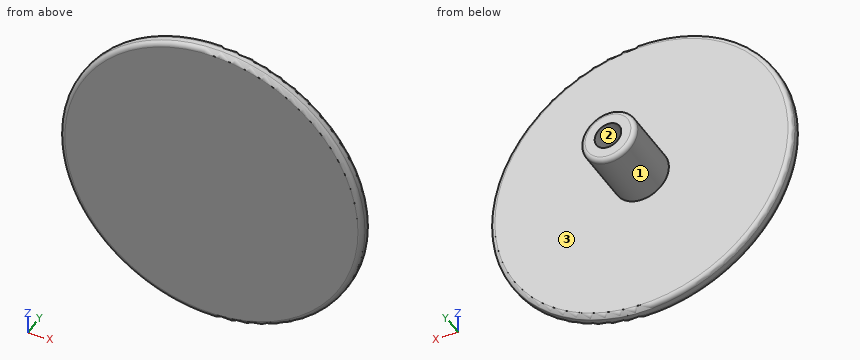
Autodesk Fusion 360 part; units mm, degrees
sketch "Sketch1" plane through (0, 0, 0) normal (0, 1, 0) x (1, 0, 0)
  circle A0 centre (0, 0) radius 16.5
  dimension "d1" = 33
extrude "Extrude1" add sketch "Sketch1" along normal blind 1.5
sketch "Sketch2" plane through (0, 1.5, 0) normal (0, 1, 0) x (-1, 0, 0)
  circle A0 centre (0, 0) radius 16.5
  circle A1 centre (0, 0) radius 3
  circle A2 centre (0, 0) radius 1.45
  dimension "d4" = 6
  dimension "d5" = 2.9
extrude "Extrude2" add sketch "Sketch2" along normal blind 7 contours A1
fillet "Fillet1" radius 0.5 3 edges at (-15.3834, 0, 5.9667) (-15.3834, 1.5, 5.9667) (2.797, 8.5, -1.0848)
The listing builds one solid part. Answer for the finished solid, in the listing's coordinates (mm). Face numbers are marked on the shaded views. Round coordinates to 2 decimals unless told otherwise and drop trailing zeros. Loops run counter-clockwise (first coordinate to the right, second up) from the corner with the lowest first, then second, coordinate; pieces in that order, holes last. Notation, with made-up numbers: (-25.5, 67) - (-20.5, 67) arc R16 ccw to (-20.5, 98) - close; hole circle Ø8 at (61.25, 60). An arc over 180 degrees is marked (long way). Return JSON: item names as keys, results as strings. Group by question number.
1. The part is cut by section B-B on z = 0. Determine the outline of the cut face in (x, y).
2. Each of these flat-tipped pins is pushed along its axis until it touches: P1, Ø5, axis at x = -3, y = 5, coming from the +Z side; P2, Ø2, axis at x = -9, z = 2, coming from the +Y side; P3, Ø1, axis at x = -3, z = -5, coming from the -Y side; P4, Ø2, axis at y = 1, z = -4.5, coming from the +X side. Where does it stop, or does it pass through?
3. Consider probe 1 along Z at (x, y) = (0, 5.5); probe 2 along Y at (x, z) = (9.5, 7.5); probe 3 along X at (y, z) = (8, -2). Determine where each line is inside the solid, lowest interval first.
4. The part is cut by section C-C on y = 2. Determine the outline of the cut face in (x, z).
5. The mould has two halves that part along X. Classify the marked faces 1, 2 and 3: pulls with the +X half, pulls with the -X half, needs draft (parallel to the pull), parting line crosses it, or undercut.
6. The part is cut by section A-A on x = 0. Determine the outline of the cut face in (y, z).
Resolved:
{
 "1": {"outline": "(-16.5, 0.5) arc R0.5 ccw to (-16, 0) - (16, 0) arc R0.5 ccw to (16.5, 0.5) - (16.5, 1) arc R0.5 ccw to (16, 1.5) - (3, 1.5) - (3, 8) arc R0.5 ccw to (2.5, 8.5) - (1.45, 8.5) - (1.45, 1.5) - (-1.45, 1.5) - (-1.45, 8.5) - (-2.5, 8.5) arc R0.5 ccw to (-3, 8) - (-3, 1.5) - (-16, 1.5) arc R0.5 ccw to (-16.5, 1) - close"},
 "2": {"P1": "stops at z = 2.96", "P2": "stops at y = 1.5", "P3": "stops at y = 0", "P4": "stops at x = 16.12"},
 "3": {"probe 1": "z = -3 to -1.45, 1.45 to 3", "probe 2": "y = 0 to 1.5", "probe 3": "x = -2.24 to 2.24"},
 "4": {"outline": "circle Ø6 at (0, 0); hole circle Ø2.9 at (0, 0)"},
 "5": {"face 1": "parting line crosses it", "face 2": "undercut", "face 3": "needs draft"},
 "6": {"outline": "(0, -16) arc R0.5 ccw to (0.5, -16.5) - (1, -16.5) arc R0.5 ccw to (1.5, -16) - (1.5, -3) - (8, -3) arc R0.5 ccw to (8.5, -2.5) - (8.5, -1.45) - (1.5, -1.45) - (1.5, 1.45) - (8.5, 1.45) - (8.5, 2.5) arc R0.5 ccw to (8, 3) - (1.5, 3) - (1.5, 16) arc R0.5 ccw to (1, 16.5) - (0.5, 16.5) arc R0.5 ccw to (0, 16) - close"}
}
